```python
from build123d import *

# Parameters (mm, degrees)
F1_DEPTH = 0.3
F2_R     = 2.75
F3_DEPTH = 6.1


with BuildPart() as f1:
    # F0 (on Top) → F1 (new body)
    with BuildSketch(Plane.XY):
        Polygon((-2.75, -2.75), (2.75, -2.75), (2.75, 1.75), (1.75, 2.75), (-1.75, 2.75), (-2.75, 1.75), align=None)
    extrude(amount=F1_DEPTH)

    # F2 (on Top) → F3 (join)
    with BuildSketch(Plane.XY):
        Circle(F2_R)
    extrude(amount=F3_DEPTH)


solid = f1.part
```
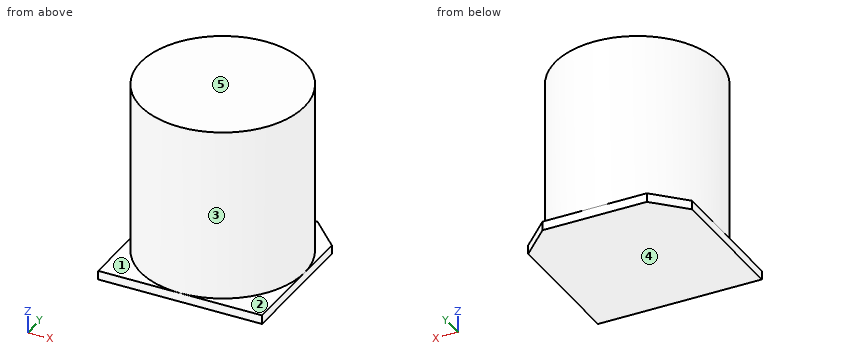
Geometry: final body of the model. Coordinates: model frame, mm. Face numbers are marked on the shaded views. A direction names the side the tool comes from. Coordinates: 2 decimals unless noted, no trailing zeros. Order: outer loops, then holes, each group sorted by start corner. A loop starts at its lowest first (then second) coordinate and runs counter-clockwise, first axis right, second up. Notation, with made-up numbers: (-31.75, 74) - (1.25, 74) arc R8 cw to (1.25, 79) - close; hole circle Ø1 at (70.25, 61). An arc over 180 degrees is marked (long way). Write each question's results on one line, items separated by ' | '.
1) Line query: line 1 (Z direction, x = 2.5, y = -2); line 2 (Y direction, x = -0.3, z = 0.5); line 3 (Y direction, x = -1.1, z = 0.5). Output: solid intervals per line, ascending. Write a range as from..to.
Results list:
line 1: 0..0.3 | line 2: -2.73..2.73 | line 3: -2.52..2.52
2) Section A-A, the plane x = 1.5. Return loops of the section in (y, z), plus the area to 3 significant figures.
Results list:
outline: (-2.75, 0) - (2.75, 0) - (2.75, 0.3) - (2.3, 0.3) - (2.3, 6.1) - (-2.3, 6.1) - (-2.3, 0.3) - (-2.75, 0.3) - close | area: 28.4 mm^2
3) Section C-C, the plane y = -0.6. Return loops of the section in (x, z), plus the area to 3 significant figures.
Results list:
outline: (-2.75, 0) - (2.75, 0) - (2.75, 0.3) - (2.68, 0.3) - (2.68, 6.1) - (-2.68, 6.1) - (-2.68, 0.3) - (-2.75, 0.3) - close | area: 32.8 mm^2
4) Set-up query: the marked faces 1 and 2. Return all of +Z, -Z, +X, -X, +Y, -Y with unobstructed straight access to the full face (end or side cutting, diameter ignored); none if empty.
Results list:
face 1: +Z, -X, -Y | face 2: +Z, +X, -Y
5) Pull-direction query (Z, two-part tool) for the marked faces 3, 4 and 5; classes: pulls with the +Z half, pulls with the -Z half, needs draft (parallel to the pull), parting line crosses it, or undercut.
Results list:
face 3: needs draft | face 4: pulls with the -Z half | face 5: pulls with the +Z half
6) Section B-B, the plane z = 4.75. Return loops of the section in (x, y), plus the area to 3 significant figures.
Results list:
outline: circle Ø5.5 at (0, 0) | area: 23.8 mm^2
